from build123d import *

# Parameters (mm, degrees)
SKETCH_R        = 20
PAD_DEPTH       = 2
SKETCH001_R     = 12.75
PAD001_DEPTH    = 18
SKETCH002_R     = 10
POCKET_DEPTH    = 20.001
CHAMFER_SIZE    = 2
CHAMFER001_SIZE = 1.99


with BuildPart() as part:
    # Sketch → Pad (new body)
    with BuildSketch(Plane.XY):
        Circle(SKETCH_R)
    extrude(amount=PAD_DEPTH)

    # Sketch001 (on Face3 of Pad) → Pad001 (join)
    with BuildSketch(Plane.XY.offset(2)):
        Circle(SKETCH001_R)
    extrude(amount=PAD001_DEPTH)

    # Sketch002 (on Face5 of Pad001) → Pocket (cut, through all)
    with BuildSketch(Plane.XY.offset(20)):
        Circle(SKETCH002_R)
    extrude(amount=-POCKET_DEPTH, mode=Mode.SUBTRACT)

    # Chamfer
    chamfer_edges = [part.edges().sort_by_distance(p)[0] for p in [
        (-12.75, 0, 20),
    ]]
    chamfer(chamfer_edges, length=CHAMFER_SIZE)

    # Chamfer001
    chamfer001_edges = [part.edges().sort_by_distance(p)[0] for p in [
        (-20, 0, 0),
    ]]
    chamfer(chamfer001_edges, length=CHAMFER001_SIZE)


solid = part.part
Read the model definition and answer for the solid it produces. Units are mm, in the model's axes. A direction names the side the tool comes from. Coordinates: 2 decimals unless noted, no trailing zeros. Loops run counter-clockwise (first coordinate to the right, second up) from the corner with the lowest first, then second, coordinate; pieces in that order, holes last.
Q1. Consider probe 1 along Y at (x, z) = (0, 8); probe 2 along Z at (x, y) = (8, 11); probe 3 along Y at (x, z) = (-3.5, 9.25). Determine where each line is inside the solid, lowest interval first.
Q2. Each of these flat-tipped pins is pushed along its axis until it touches: pin 1 Ø12 at (x, z) = (-4, 16.5) entering from -Y; pin 2 Ø2 at (x, z) = (6, 14) entering from +Y; pin 3 Ø2 at (x, z) = (7.5, 12) entering from -Y. Where does it stop, or does it pass through?
Q3. The mould has two halves that part along X. Classify faces 3 (the face through (-2.17, -9.76, 10.14)), 4 (the face through (-2.764, -12.447, 9.888)), 5 (the face through (3, -10, 20)): +X half, -X half, draft (parallel to the pull), parting line (faces both ways), or undercut.
Q4. The part is cut by section C-C on z = 8. Write down the section's boundary in (x, y).
Q5. Which of the six approach directions +Z, -Z, +X, -X, +Y, -Y give full straight-line access (tool end or side, diameter ignored) to faces 1 (the face through (0, -13, 2)), 2 (the face through (8, -8, 0))?
Results below:
1. probe 1: y = -12.75 to -10, 10 to 12.75
1. probe 2: z = 0 to 2
1. probe 3: y = -12.26 to -9.37, 9.37 to 12.26
2. pin 1: stops at y = -12.75
2. pin 2: stops at y = 11.73
2. pin 3: stops at y = -10.97
3. face 3: undercut
3. face 4: parting line
3. face 5: draft
4. outline: circle Ø25.5 at (0, 0); hole circle Ø20 at (0, 0)
5. face 1: +Z
5. face 2: -Z, +X, -X, +Y, -Y
